```python
from build123d import *

# Parameters (mm, degrees)
BOSS_EXTRUDE1_DEPTH = 50
SKETCH2_R           = 2.545489134
CUT_EXTRUDE1_DEPTH  = 50


with BuildPart() as part:
    # Sketch1 → Boss-Extrude1 (new body)
    with BuildSketch(Plane.XY):
        with BuildLine():
            Line((-9.516237222, -14.74726776), (8.035250311, -14.74726776))
            Line((8.035250311, -14.74726776), (8.035250311, -25.75856102))
            Line((8.035250311, -25.75856102), (-10.447991948, -25.75856102))
            ThreePointArc((-10.447991948, -25.75856102), (-22.639066629, -13.567486339), (-34.83014131, -25.75856102))
            Line((-34.83014131, -25.75856102), (-54.49316499, -25.75856102))
            Line((-54.49316499, -25.75856102), (-54.49316499, -14.74726776))
            Line((-54.49316499, -14.74726776), (-35.761896036, -14.74726776))
            ThreePointArc((-35.761896036, -14.74726776), (-22.639066629, -5.330023584), (-9.516237222, -14.74726776))
        make_face()
    extrude(amount=BOSS_EXTRUDE1_DEPTH)

    # Sketch2 → Cut-Extrude1 (cut)
    with BuildSketch(Plane(origin=(0, 0, 0), x_dir=(1, 0, 0), z_dir=(0, 1, 0))):
        with Locations((-47.57711427, -10.003748799)):
            Circle(SKETCH2_R)
        with Locations((0, -10.003748799)):
            Circle(SKETCH2_R)
        with Locations((0, -39.664230879)):
            Circle(SKETCH2_R)
        with Locations((-47.57711427, -39.664230879)):
            Circle(SKETCH2_R)
    extrude(amount=-CUT_EXTRUDE1_DEPTH, mode=Mode.SUBTRACT)


solid = part.part
```
Work out the finished part from the listing and answer in its coordinate system (mm). A direction names the side the tool comes from. Coordinates: 2 decimals unless noted, no trailing zeros. Loops run counter-clockwise (first coordinate to the right, second up) from the corner with the lowest first, then second, coordinate; pieces in that order, holes last.
1) Consider probe 1 along Z at (x, y) = (0, -17.5); probe 2 along Y at (x, z) = (-43, 9); probe 3 along X at (y, z) = (-19.5, 28.5). Determine where each line is inside the solid, lowest interval first.
Results:
probe 1: z = 0 to 7.46, 12.55 to 37.12, 42.21 to 50
probe 2: y = -25.76 to -14.75
probe 3: x = -54.49 to -33.1, -12.18 to 8.04
2) Section A-A (x = 0) is taken. Give the vertices of the cut face in (y, z), plus the area to 3 significant figures.
Results:
outline: (-25.76, 0) - (-14.75, 0) - (-14.75, 7.46) - (-25.76, 7.46) - close; (-25.76, 12.55) - (-14.75, 12.55) - (-14.75, 37.12) - (-25.76, 37.12) - close; (-25.76, 42.21) - (-14.75, 42.21) - (-14.75, 50) - (-25.76, 50) - close
area: 438 mm2
3) Section C-C (z = 17) is taken. Give the vertices of the cut face in (x, y).
Results:
outline: (-54.49, -25.76) - (-34.83, -25.76) arc R12.19 cw to (-10.45, -25.76) - (8.04, -25.76) - (8.04, -14.75) - (-9.52, -14.75) arc R13.85 ccw to (-35.76, -14.75) - (-54.49, -14.75) - close
4) For a pull along Z with two mould halves and no side action, classify faces 4 (the flat face through (-23, -13, 50)), 5 (the cylindrical face through (-50.12, -20.18, 39.55)), 6 (the cylindrical face through (-22.88, -5.332, 24.65)) as +Z half, -Z half, draft (parallel to the pull), parting line (faces both ways), or undercut.
Results:
face 4: +Z half
face 5: undercut
face 6: draft
5) Flat-ended cylindrical pins translate along their axes: pin 1 (6.5 mm diameter, centred on x = -47.58, z = 10, fed in from +Y); pin 2 (4 mm diameter, centred on y = -13, z = 30, fed in from -X); pin 3 (3 mm diameter, centred on x = -16.5, z = 15.5, fed in from +Y); pin 4 (19.5 mm diameter, centred on x = -1, z = 33, fed in from +Y). Find the tip coordinate at first contact, or state that the pin passes through.
Results:
pin 1: stops at y = -14.75
pin 2: stops at x = -54.49
pin 3: stops at y = -6.13
pin 4: stops at y = -12.07
6) Section D-D (x = -16.5) is taken. Give the vertices of the cut face in (y, z), plus the area to 3 significant figures.
Results:
outline: (-15.23, 0) - (-6.76, 0) - (-6.76, 50) - (-15.23, 50) - close
area: 423 mm2
7) Section B-B (y = -21.75) is taken. Give the vertices of the cut face in (x, z).
Results:
outline: (-54.49, 0) - (-34.15, 0) - (-34.15, 50) - (-54.49, 50) - close; (-11.13, 0) - (8.04, 0) - (8.04, 50) - (-11.13, 50) - close; hole circle Ø5.09 at (-47.58, 10); hole circle Ø5.09 at (-47.58, 39.66); hole circle Ø5.09 at (0, 10); hole circle Ø5.09 at (0, 39.66)
8) For faces 1 (the flat face through (-45, -14.747, 25)), 2 (the flat face through (-1, -14.747, 25)), 3 (the cylindrical face through (-2.02, -20.18, 11.55)), determine the directions among +Z, -Z, +X, -X, +Y, -Y from which every point of the face is accessible in a straight line to the end or side of a thin tool.
Results:
face 1: +Z, -Z, -X, +Y
face 2: +Z, -Z, +X, +Y
face 3: +Y, -Y
